Verification items for this drawing (mm, ordinates from the low corner). A direction names the side the tool comes from. Coordinates: 2 decimals unless noted, no trailing zeros. Loops run counter-clockwise (first coordinate to the right, second up) from the corner with the lowest first, then second, coordinate; pieces in that order, holes last. Notation, with made-up numbers: (3, 11.25) -> (26, 11.25) arc R24 cw to (26, 43.25) -> close; hole circle Ø8 at (36.25, -1.75). An arc over 180 degrees is marked (long way). Write item = value, one per line.
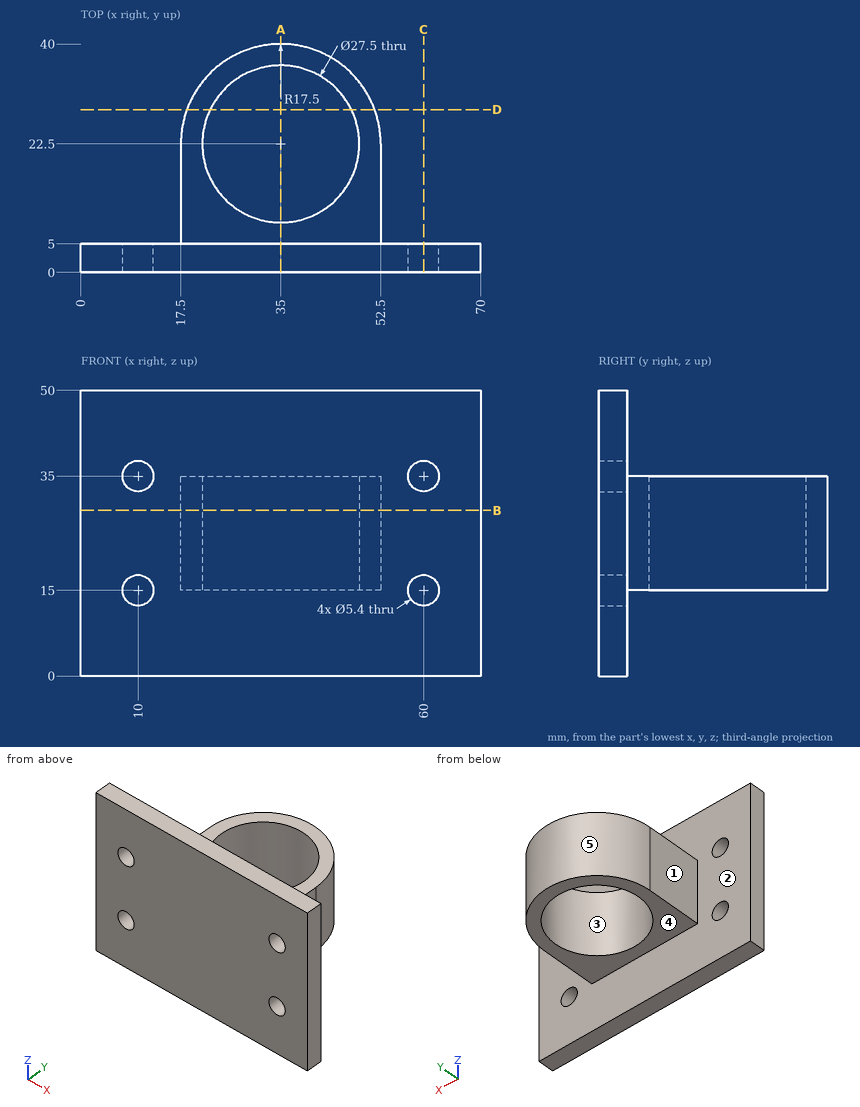
1) Tool access check on the marked faces 4 and 5. Record the directions out of +Z, -Z, +X, -X, +Y, -Y that give a thin tool (end or side, any length) a straight path to the whole face; none if there is none.
Ans:
face_4 = -Z, +X, -X, +Y
face_5 = +Z, -Z, +Y
2) Sectioned sample at B-B, the plane z = 29. Record the cut outline in (x, y), plus the area to 3 significant figures.
Ans:
outline = (0, 0) -> (70, 0) -> (70, 5) -> (52.5, 5) -> (52.5, 22.5) arc R17.5 ccw to (17.5, 22.5) -> (17.5, 5) -> (0, 5) -> close; hole circle Ø27.5 at (35, 22.5)
area = 850 mm2
3) Sectioned sample at A-A, the plane x = 35. Record the cut outline in (y, z).
Ans:
outline = (0, 0) -> (5, 0) -> (5, 15) -> (8.75, 15) -> (8.75, 35) -> (5, 35) -> (5, 50) -> (0, 50) -> close; (36.25, 15) -> (40, 15) -> (40, 35) -> (36.25, 35) -> close
4) Sectioned sample at D-D, the plane y = 28.5. Record the cut outline in (x, z), plus the area to 3 significant figures.
Ans:
outline = (18.56, 15) -> (22.63, 15) -> (22.63, 35) -> (18.56, 35) -> close; (47.37, 15) -> (51.44, 15) -> (51.44, 35) -> (47.37, 35) -> close
area = 163 mm2
5) Release check for a two-part mould opening along X. For the marked faces 1, 2 and 3 record: pulls with the +X half, pulls with the -X half, needs draft (parallel to the pull), parting line crosses it, or undercut.
Ans:
face_1 = pulls with the -X half
face_2 = needs draft
face_3 = undercut
6) Depth check by flat-ended pin: pin 1 Ø10.5 at (x, y) = (28, 19) entering from +Z; pin 2 Ø1 at (x, z) = (13, 35.5) entering from +Y; pin 3 Ø9 at (y, z) = (15, 24.5) entering from -X; pin 4 Ø14 at (y, z) = (17.5, 25.5) entering from +X. Enter the tip coordinate at first touch or a pass-through.
Ans:
pin_1 = through
pin_2 = 5
pin_3 = 17.5
pin_4 = 52.5
7) Material ranges on line 1 (X direction, y = 1.8, z = 35); line 2 (Z direction, x = 10, y = 3); line 3 (Y direction, x = 35, z = 20.5), recorded low to high.
Ans:
line_1 = 0 to 7.3, 12.7 to 57.3, 62.7 to 70
line_2 = 0 to 12.3, 17.7 to 32.3, 37.7 to 50
line_3 = 0 to 8.75, 36.25 to 40
8) Sectioned sample at C-C, the plane x = 60. Record the cut outline in (y, z), plus the area to 3 significant figures.
Ans:
outline = (0, 0) -> (5, 0) -> (5, 12.3) -> (0, 12.3) -> close; (0, 17.7) -> (5, 17.7) -> (5, 32.3) -> (0, 32.3) -> close; (0, 37.7) -> (5, 37.7) -> (5, 50) -> (0, 50) -> close
area = 196 mm2
